Autodesk Inventor part; units mm, degrees
ref_plane "YZ Plane" through (0, 0, 0) normal (1, 0, 0) x (0, 1, 0)
ref_plane "XZ Plane" through (0, 0, 0) normal (0, 1, 0) x (-1, 0, 0)
ref_plane "XY Plane" through (0, 0, 0) normal (0, 0, 1) x (1, 0, 0)
sketch "Sketch1" plane through (0, 0, 0) normal (0, 0, 1) x (1, 0, 0)
  line L0 (-63.5, -63.5) -> (63.5, -63.5)
  line L1 (63.5, -63.5) -> (63.5, 63.5)
  line L2 (63.5, 63.5) -> (-63.5, 63.5)
  line L3 (-63.5, 63.5) -> (-63.5, -63.5)
  line L4 (-63.5, -63.5) -> (63.5, 63.5) construction
  line L5 (63.5, -63.5) -> (-63.5, 63.5) construction
  line L6 (-69.85, -69.85) -> (69.85, -69.85)
  line L7 (69.85, -69.85) -> (69.85, 69.85)
  line L8 (69.85, 69.85) -> (-69.85, 69.85)
  line L9 (-69.85, 69.85) -> (-69.85, -69.85)
  line L10 (-57.15, -57.15) -> (57.15, -57.15)
  line L11 (57.15, -57.15) -> (57.15, 57.15)
  line L12 (57.15, 57.15) -> (-57.15, 57.15)
  line L13 (-57.15, 57.15) -> (-57.15, -57.15)
  point P0 (0, 0)
  dimension "d0" = 127
  dimension "d1" = 127
  dimension "d2" = 6.35
  dimension "d3" = 6.35
extrude "Extrusion1" add sketch "Sketch1" along normal blind 5.08 contours L3 L2 L1 L0 | L9 L8 L7 L6
sketch "Sketch2" plane through (0, 0, 5.08) normal (0, 0, 1) x (1, 0, 0)
  line L0 (-57.15, -57.15) -> (-57.15, 57.15)
  line L1 (-57.15, 57.15) -> (57.15, 57.15)
  line L2 (57.15, 57.15) -> (57.15, -57.15)
  line L3 (57.15, -57.15) -> (-57.15, -57.15)
  line L4 (-69.85, -69.85) -> (69.85, -69.85)
  line L5 (69.85, -69.85) -> (69.85, 69.85)
  line L6 (69.85, 69.85) -> (-69.85, 69.85)
  line L7 (-69.85, 69.85) -> (-69.85, -69.85)
  point P0 (0, 0)
  point P1 (-66.675, 66.675)
  dimension "d6" = 3.175
  dimension "d7" = 3.175
hole "Hole1" at (-66.675, 66.675, 5.08) direction (0, 0, -1) diameter 3.264 end through all
mirror "Mirror1" about plane through (0, 0, 0) normal (0, 1, 0) of "Hole1"
mirror "Mirror2" about plane through (0, 0, 0) normal (1, 0, 0) of "Hole1", "Mirror1"
fillet "Fillet1" radius 6.35 4 edges at (-57.15, 57.15, 2.54) (57.15, 57.15, 2.54) (-57.15, -57.15, 2.54) (57.15, -57.15, 2.54)
properties part number "spacer" material "Aluminum 6061"
Part model, mm, in its own coordinate system. A direction names the side the tool comes from. Give positions to 0.01 mm unless a question says otherwise; leave off trailing zeros. Write each loop counter-clockwise with the first axis right and the second up, starting at its lowest first coordinate (ties: lowest second). Pieces come first, ordered by that corner, then holes.
1) Pin check, flat tips, straight feed: pin 1 (4 mm diameter, centred on x = -66.675, y = 66.675, fed in from -Z); pin 2 (2 mm diameter, centred on x = 66.675, y = 66.675, fed in from -Z). Stop position of each tip, or through.
Resolved:
pin 1: stops at z = 0
pin 2: passes through
2) Two-plate mould, pull along X, no slides. Class faces 1 (the face through (-69.85, 1, 3)), 2 (the face through (-1, -57.15, 3)), 3 (the face through (1, 69.85, 3)): released by +X, released by -X, zero draft, split by the parting line, or undercut.
Resolved:
face 1: released by -X
face 2: undercut
face 3: zero draft
3) Probe L1, parallel to Y at x = -28.5, z = 0.8; L2, parallel to Y at x = 53.5, z = 2.05. List the from-to ranges inside material, lowest first.
Resolved:
L1: y = -69.85 to -57.15, 57.15 to 69.85
L2: y = -69.85 to -56.55, 56.55 to 69.85
4) Cut at C-C on z = 3.2. Write the cut outline in (x, y) (3 decimals), then the cut area to 3 significant figures.
Resolved:
outline: (-69.85, -69.85) - (69.85, -69.85) - (69.85, 69.85) - (-69.85, 69.85) - close; hole circle Ø3.264 at (-66.675, -66.675); hole circle Ø3.264 at (-66.675, 66.675); hole (-57.15, -50.8) arc R6.35 ccw to (-50.8, -57.15) - (50.8, -57.15) arc R6.35 ccw to (57.15, -50.8) - (57.15, 50.8) arc R6.35 ccw to (50.8, 57.15) - (-50.8, 57.15) arc R6.35 ccw to (-57.15, 50.8) - close; hole circle Ø3.264 at (66.675, -66.675); hole circle Ø3.264 at (66.675, 66.675)
area: 6,450 mm2
5) Which spindle directions (+Z, -Z, +X, -X, +Y, -Y) get a long thin tool onto all of the face, cutting with end or side? Do faces 4 (the face through (-55.24, 55.34, 2.58)), 5 (the face through (69.85, -1, 3)). Say none if no direction does.
Resolved:
face 4: +Z, -Z
face 5: +Z, -Z, +X, +Y, -Y
6) Cut at A-A on y = 47. Write the cut outline in (x, z), then the cut area to 3 significant figures.
Resolved:
outline: (-69.85, 0) - (-57.15, 0) - (-57.15, 5.08) - (-69.85, 5.08) - close; (57.15, 0) - (69.85, 0) - (69.85, 5.08) - (57.15, 5.08) - close
area: 129 mm2
